Can you work these out from the drawing? Everything is in mm from the part's minimum corner. A direction names the side the tool comes from. Give positions to 0.01 mm unless a question says otherwise; leave off trailing zeros. Order: outer loops, then holes, each group sorted by start corner. A loop starts at its lowest first (then second) coordinate and runs counter-clockwise, first axis right, second up. Notation, with made-up numbers: (-0.75, 26) - (29.25, 26) arc R23 cw to (29.25, 47) - close; hole circle Ø4 at (48.5, 56.5). An arc over 180 degrees is marked (long way). One line per question, with ' | ' between items.
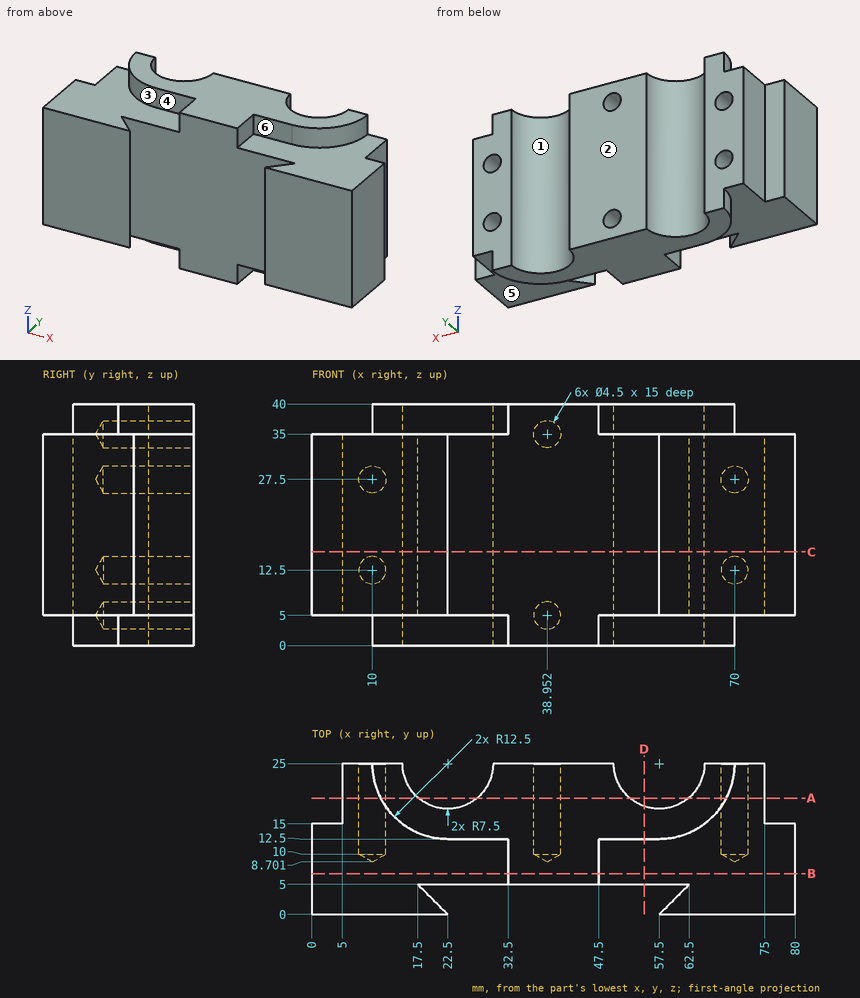
(1) If we mould it in two halves opening along X, with no side actions, what happens to the marked faces 1, 2 and 3? For each: released by +X, released by -X, zero draft, split by the parting line, or undercut.
Answer below:
face 1: undercut | face 2: zero draft | face 3: released by -X
(2) Imagine slicing it at B-B (y = 6.75). List the corners of the cut face in (x, z) for me, and give its area (3 significant figures).
Answer below:
outline: (0, 5) - (32.5, 5) - (32.5, 0) - (47.5, 0) - (47.5, 5) - (80, 5) - (80, 35) - (47.5, 35) - (47.5, 40) - (32.5, 40) - (32.5, 35) - (0, 35) - close | area: 2,550 mm^2
(3) Will these pins go through, and if not, where does the flat tip stop? pin 1 (2.5 mm diameter, centred on x = 70, z = 27.5, fed in from +Y); pin 2 (1.5 mm diameter, centred on x = 78, z = 24, fed in from +Y); pin 3 (3.5 mm diameter, centred on x = 38.95, z = 35, fed in from +Y).
Answer below:
pin 1: y = 9.42 | pin 2: y = 15 | pin 3: y = 9.71
(4) Imagine slicing it at D-D (x = 55). List the corners of the cut face in (y, z) for me, and give its area (3 significant figures).
Answer below:
outline: (5, 5) - (12.5, 5) - (12.5, 0) - (17.93, 0) - (17.93, 40) - (12.5, 40) - (12.5, 35) - (5, 35) - close | area: 442 mm^2
(5) Imagine slicing it at C-C (z = 15.5). List the corners of the cut face in (x, y) for me, and give its area (3 significant figures).
Answer below:
outline: (0, 0) - (22.5, 0) - (17.5, 5) - (62.5, 5) - (57.5, 0) - (80, 0) - (80, 15) - (75, 15) - (75, 25) - (65, 25) arc R7.5 cw to (50, 25) - (30, 25) arc R7.5 cw to (15, 25) - (5, 25) - (5, 15) - (0, 15) - close | area: 1,520 mm^2
(6) If I drill on line 1 (X direction, y = 14, z = 27.5); line 2 (Z direction, x = 70, y = 16.5); line 3 (Z direction, x = 8, y = 15.25), over which ranges is the centre line in solid material (lowest first)?
Answer below:
line 1: 0 to 7.75, 12.25 to 67.75, 72.25 to 80 | line 2: 5 to 10.25, 14.75 to 25.25, 29.75 to 35 | line 3: 5 to 11.47, 13.53 to 26.47, 28.53 to 35
(7) Imagine slicing it at A-A (y = 19.25). Count the separate pieces of the cut face and the enclosed holes in it, and give its area (3 significant figures).
Answer below:
separate pieces: 3 | enclosed holes: 6 | area: 1,810 mm^2
(8) On a 3-axis mill with a long thin cutter (end or side, diameter ignored), from which of +Z, -Z, +X, -X, +Y, -Y can I reach the whole of each face in a straight line? I mean the marked faces 4, 5 and 6. Say none if no direction works.
Answer below:
face 4: +Z, -X, -Y | face 5: -Z, +X, -Y | face 6: +Z, +X, -Y
